The model under review builds one solid part; all positions refer to its coordinate system, in mm. A direction names the side the tool comes from. Coordinates: 2 decimals unless noted, no trailing zeros. Write each loop counter-clockwise with the first axis right and the second up, starting at its lowest first coordinate (ties: lowest second). Pieces come first, ordered by that corner, then holes.
```python
from build123d import *

# Parameters (mm, degrees)
SKETCH_1_R      = 2
EXTRUDE_1_DEPTH = 21


with BuildPart() as part:
    # 草图1 → 凸台-拉伸1 (new body)
    with BuildSketch(Plane.XY):
        with BuildLine():
            Line((-21, 18), (-18, 21))
            Line((-18, 21), (-10, 21))
            Line((-10, 21), (-10, 11.180339887))
            ThreePointArc((-10, 11.180339887), (0, -15), (10, 11.180339887))
            Line((10, 11.180339887), (10, 21))
            Line((10, 21), (18, 21))
            Line((18, 21), (21, 18))
            Line((21, 18), (21, -18))
            Line((21, -18), (18, -21))
            Line((18, -21), (-18, -21))
            Line((-18, -21), (-21, -18))
            Line((-21, -18), (-21, 18))
        make_face()
        with Locations(Location((15.5, 15.5, 0), (0, 0, 180))):
            Circle(SKETCH_1_R, mode=Mode.SUBTRACT)
        with Locations(Location((15.5, -15.5, 0), (0, 0, 180))):
            Circle(SKETCH_1_R, mode=Mode.SUBTRACT)
        with Locations(Location((-15.5, -15.5, 0), (0, 0, 180))):
            Circle(SKETCH_1_R, mode=Mode.SUBTRACT)
        with Locations(Location((-15.5, 15.5, 0), (0, 0, 180))):
            Circle(SKETCH_1_R, mode=Mode.SUBTRACT)
    extrude(amount=EXTRUDE_1_DEPTH)


solid = part.part
```
Item 1: Take a section at B-B, the plane y = 0. Write out the cut boundary in (x, z), plus the area to 3 significant figures.
Solved:
outline: (-21, 0) - (-15, 0) - (-15, 21) - (-21, 21) - close; (15, 0) - (21, 0) - (21, 21) - (15, 21) - close
area: 252 mm2
Item 2: For pin 1 (3.5 mm diameter, centred on x = -15.5, y = -15.5, fed in from -Z); pin 2 (6.5 mm diameter, centred on x = 15.5, y = 15.5, fed in from -Z), all flat-tipped, find the tip position at first contact; note any pin that passes through.
Solved:
pin 1: passes through
pin 2: stops at z = 0
Item 3: To check wall thickness, follow line 1 along Y through (x, z) = (15.5, 6.75); line 2 along X through (y, z) = (15.5, 12). State the ranges of each line that lie inside material, in increasing order.
Solved:
line 1: y = -21 to -17.5, -13.5 to 13.5, 17.5 to 21
line 2: x = -21 to -17.5, -13.5 to -10, 10 to 13.5, 17.5 to 21
Item 4: Mouldability with a two-part tool opening along Y and no side actions: class faces 3 (the face through (-9, -14, 21)), 4 (the face through (0, -21, 10)), 5 (the face through (19, 20, 10)), 6 (the face through (-0.51, -14.99, 10.35)) as pulls with the +Y half, pulls with the -Y half, needs draft (parallel to the pull), parting line crosses it, or undercut.
Solved:
face 3: needs draft
face 4: pulls with the -Y half
face 5: pulls with the +Y half
face 6: undercut
Item 5: Machinability: for faces 1 (the face through (-15.24, 13.517, 10.353)), 2 (the face through (-10, 16, 10)), which of the approach directions +Z, -Z, +X, -X, +Y, -Y give a long, thin tool a straight path to every point of the face, cutting with its end or side? Answer none if there is none.
Solved:
face 1: +Z, -Z
face 2: +Z, -Z, +Y
Item 6: Take a section at A-A, the plane y = 15.5. Write out the cut boundary in (x, z).
Solved:
outline: (-21, 0) - (-17.5, 0) - (-17.5, 21) - (-21, 21) - close; (-13.5, 0) - (-10, 0) - (-10, 21) - (-13.5, 21) - close; (10, 0) - (13.5, 0) - (13.5, 21) - (10, 21) - close; (17.5, 0) - (21, 0) - (21, 21) - (17.5, 21) - close
Item 7: Take a section at C-C, the plane z = 17. Write out the cut boundary in (x, y).
Solved:
outline: (-21, -18) - (-18, -21) - (18, -21) - (21, -18) - (21, 18) - (18, 21) - (10, 21) - (10, 11.18) arc R15 cw (long way) to (-10, 11.18) - (-10, 21) - (-18, 21) - (-21, 18) - close; hole circle Ø4 at (-15.5, -15.5); hole circle Ø4 at (-15.5, 15.5); hole circle Ø4 at (15.5, -15.5); hole circle Ø4 at (15.5, 15.5)
Item 8: Take a section at D-D, the plane x = 0. Write out the cut boundary in (y, z), plus the area to 3 significant figures.
Solved:
outline: (-21, 0) - (-15, 0) - (-15, 21) - (-21, 21) - close
area: 126 mm2
